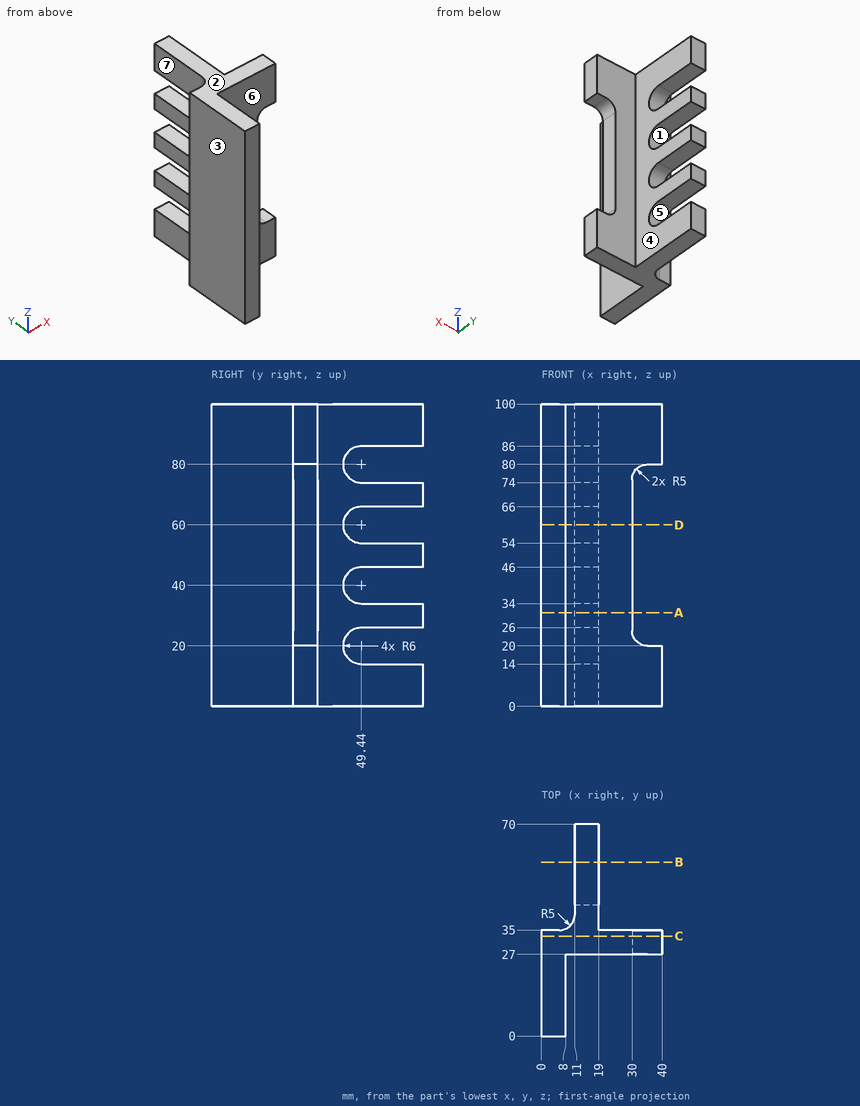
Source: three-view drawing plus pictorial views. Frame: mm from the lowest corner of the part. A direction names the side the tool comes from. Coordinates: 2 decimals unless noted, no trailing zeros. Loops run counter-clockwise (first coordinate to the right, second up) from the corner with the lowest first, then second, coordinate; pieces in that order, holes last. Notation, with made-up numbers: (27, -1.5) -> (38, -1.5) arc R6 ccw to (38, 8.5) -> close; hole circle Ø11 at (42, -40). An arc over 180 degrees is marked (long way). One line per item, written item: value.
(1) Ray query, line 1 along Z through (x, y) = (13.5, 57.5); line 2 along Y through (x, z) = (29, 29.5); line 3 along Y through (x, z) = (14.5, 39.5). Return the intervals inside material, ascending.
Answer below:
line 1: z = 0 to 14, 26 to 34, 46 to 54, 66 to 74, 86 to 100
line 2: y = 27 to 35
line 3: y = 27 to 43.46
(2) Cut plane A-A (z = 31). Output: boundary loops of the cut face in (x, y), then the cut area to 3 significant figures.
Answer below:
outline: (0, 0) -> (8, 0) -> (8, 27) -> (30, 27) -> (30, 35) -> (19, 35) -> (19, 70) -> (11, 70) -> (11, 40) arc R5 cw to (6, 35) -> (0, 35) -> close
area: 741 mm2
(3) Cut plane C-C (y = 33). Output: boundary loops of the cut face in (x, z), then the cut area to 3 significant figures.
Answer below:
outline: (0, 0) -> (40, 0) -> (40, 20) -> (35, 20) arc R5 cw to (30, 25) -> (30, 75) arc R5 cw to (35, 80) -> (40, 80) -> (40, 100) -> (0, 100) -> close
area: 3,410 mm2
(4) Draft query along Z for the marked faces 1, 2 and 3. Return one class per face: pulls with the +Z half, pulls with the -Z half, needs draft (parallel to the pull), parting line crosses it, or undercut.
Answer below:
face 1: undercut
face 2: pulls with the +Z half
face 3: needs draft
(5) Pin query (flat end, axial travel): pin 1 Ø1.5 at (y, z) = (59.5, 49.5) entering from -X; pin 2 Ø8 at (y, z) = (33, 33.5) entering from +X; pin 3 Ø12 at (x, z) = (26, 46) entering from -Y. Return the tip coordinate at first contact, or that it passes through.
Answer below:
pin 1: stops at x = 11
pin 2: stops at x = 30
pin 3: stops at y = 27
(6) Cut plane B-B (y = 57.5). Output: boundary loops of the cut face in (x, z).
Answer below:
outline: (11, 0) -> (19, 0) -> (19, 14) -> (11, 14) -> close; (11, 26) -> (19, 26) -> (19, 34) -> (11, 34) -> close; (11, 46) -> (19, 46) -> (19, 54) -> (11, 54) -> close; (11, 66) -> (19, 66) -> (19, 74) -> (11, 74) -> close; (11, 86) -> (19, 86) -> (19, 100) -> (11, 100) -> close
(7) Set-up query: the marked faces 4, 5, 6 and 7. Return all of +Z, -Z, +X, -X, +Y, -Y with unobstructed straight access to the full face (end or side cutting, diameter ignored); none if empty.
Answer below:
face 4: +Z, -Z, +X, +Y
face 5: +X, -X, +Y
face 6: +Z, -Z, +X, -Y
face 7: +Z, -Z, -X, +Y
(8) Cut plane D-D (z = 60). Output: boundary loops of the cut face in (x, y).
Answer below:
outline: (0, 0) -> (8, 0) -> (8, 27) -> (30, 27) -> (30, 35) -> (19, 35) -> (19, 43.44) -> (11, 43.44) -> (11, 40) arc R5 cw to (6, 35) -> (0, 35) -> close
